Geometry: final body of the model. Coordinates: model frame, mm. Face numbers are marked on the shaded views. A direction names the side the tool comes from. Coordinates: 2 decimals unless noted, no trailing zeros. Order: outer loops, then holes, each group sorted by start corner. A loop starts at its lowest first (then second) coordinate and runs counter-clockwise, first axis right, second up. Notation, with made-up numbers: M 32,68.5 L 77,68.5 A22 cw 77,77.5 Z; hole C -25.5,62.5 d8. An arc over 180 degrees is marked long. One line per question, with ' | ' between items.
from build123d import *

# Parameters (mm, degrees)
BOSS_EXTRUDE2_DEPTH             = 2.1082
BOSS_EXTRUDE3_DEPTH             = 0.9
SKETCH13_W                      = 5.200208993
SKETCH13_H                      = 1.5
BOSS_EXTRUDE4_DEPTH             = 12.7
SKETCH16_W                      = 7.09322036
SKETCH16_H                      = 1.5
BOSS_EXTRUDE5_DEPTH             = 11.8
SKETCH17_W                      = 1.5
SKETCH17_H                      = 23.6
BOSS_EXTRUDE6_DEPTH             = 38.1
BOSS_EXTRUDE7_REACH             = 53.45
BOSS_EXTRUDE8_DEPTH             = 3.0082
CUT_EXTRUDE1_DEPTH              = 52.450131959
CUT_EXTRUDE2_REACH              = 52.338
SKETCH21_R                      = 2.794
SKETCH22_R                      = 4.572
CUT_EXTRUDE3_DEPTH              = 51.337641034
BOSS_EXTRUDE9_REACH             = 52.338
BOSS_EXTRUDE9_DIRECTION_2_DEPTH = 1.5


with BuildPart() as part:
    # Sketch6 → Boss-Extrude2 (new body)
    with BuildSketch(Plane(origin=(0, 0, 0), x_dir=(1, 0, 0), z_dir=(0, 1, 0))):
        with BuildLine():
            Line((3.1496, 3.175), (3.1496, 8.27377964))
            Line((3.1496, 8.27377964), (-5.741348421, 8.27377964))
            Line((-5.741348421, 8.27377964), (-8.59506403, 5.42006403))
            ThreePointArc((-8.59506403, 5.42006403), (-9.283317516, 4.390019898), (-9.525, 3.175))
            Line((-9.525, 3.175), (-9.525, -1.92377964))
            Line((-9.525, -1.92377964), (-6.989909723, -1.92377964))
            Line((-6.989909723, -1.92377964), (3.1496, -1.92377964))
            Line((3.1496, -1.92377964), (3.1496, 3.175))
        make_face()
    extrude(amount=BOSS_EXTRUDE2_DEPTH)

    # Sketch7 → Boss-Extrude3 (add)
    with BuildSketch(Plane.XZ):
        with BuildLine():
            Line((-2.050608993, 1.92377964), (-2.050608993, 0.42377964))
            ThreePointArc((-2.050608993, 0.42377964), (-0.881374643, -4.411978027), (-4.017957094, -8.27377964))
            Line((-4.017957094, -8.27377964), (6.35, -8.27377964))
            ThreePointArc((6.35, -8.27377964), (11.44877964, -3.175), (6.35, 1.92377964))
            Line((6.35, 1.92377964), (-2.050608993, 1.92377964))
        make_face()
    extrude(amount=BOSS_EXTRUDE3_DEPTH)

    # Sketch10 → Revolve2 (revolve)
    with BuildSketch(Plane.XY.offset(-3.175), mode=Mode.PRIVATE) as revolve2_sk:
        with BuildLine():
            Line((-6.35, 0), (-6.35, -1.065979307))
            ThreePointArc((-6.35, -1.065979307), (-5.088839039, -0.786386653), (-4.064, 0))
            Line((-4.064, 0), (-6.35, 0))
        make_face()
    revolve(revolve2_sk.sketch.rotate(Axis((-6.35, 0, -3.175), (0, -1, 0)), 180), axis=Axis((-6.35, 0, -3.175), (0, -1, 0)))

    # Sketch13 → Boss-Extrude4 (add)
    with BuildSketch(Plane.XZ):
        with Locations((0.549495504, 1.17377964)):
            Rectangle(SKETCH13_W, SKETCH13_H)
    extrude(amount=BOSS_EXTRUDE4_DEPTH)

    # Sketch16 → Boss-Extrude5 (add)
    with BuildSketch(Plane.XZ.offset(0.9)):
        with Locations((2.80338982, -7.52377964)):
            Rectangle(SKETCH16_W, SKETCH16_H)
    extrude(amount=BOSS_EXTRUDE5_DEPTH)

    # Mirror1: part across plane


with BuildPart() as part_1:
    add(part.part)
    add(part.part.mirror(Plane(origin=(3.1496, -12.7, 1.92377964), x_dir=(0, 0, 1), z_dir=(0, 1, 0))))

    # Sketch17 → Boss-Extrude6 (add)
    with BuildSketch(Plane(origin=(3.1496, 0, 0), x_dir=(0, 0, -1), z_dir=(1, 0, 0))):
        with Locations((-1.17377964, -12.7)):
            Rectangle(SKETCH17_W, SKETCH17_H)
    extrude(amount=BOSS_EXTRUDE6_DEPTH)

    # Boss-Extrude7: up to this face of the body (flat: up to its plane)
    boss_extrude7_end = Plane(part_1.part.faces().sort_by_distance((25.033512305, -24.5, 1.184664169))[0])
    # Sketch18 → Boss-Extrude7 (add, up to the picked face)
    with BuildSketch(Plane.XZ.offset(27.5082), mode=Mode.PRIVATE) as boss_extrude7_sk1:
        Polygon((3.1496, -8.27377964), (41.2496, 0.42377964), (41.2496, 1.92377964), (3.1496, 1.92377964), align=None)
    boss_extrude7_tool1 = split(extrude(boss_extrude7_sk1.sketch, amount=-BOSS_EXTRUDE7_REACH, mode=Mode.PRIVATE), bisect_by=boss_extrude7_end, keep=Keep.BOTH, mode=Mode.PRIVATE)
    add(boss_extrude7_tool1.solids().sort_by(Axis((17.478145, -27.5082, -1.539523), (0, 1, 0)))[0])

    # Sketch19 → Boss-Extrude8 (add)
    with BuildSketch(Plane(origin=(0, 2.1082, 0), x_dir=(1, 0, 0), z_dir=(0, 1, 0))):
        Polygon((3.1496, 8.27377964), (41.2496, -0.42377964), (41.2496, -1.92377964), (3.1496, -1.92377964), align=None)
    extrude(amount=-BOSS_EXTRUDE8_DEPTH)

    # Sketch20 → Cut-Extrude1 (cut, through all)
    with BuildSketch(Plane.XZ.offset(27.5082)):
        with BuildLine():
            Line((10.03132609, -6.702802721), (3.1496, -8.27377964))
            Line((3.1496, -8.27377964), (6.35, -8.27377964))
            ThreePointArc((6.35, -8.27377964), (8.351257746, -7.864618455), (10.03132609, -6.702802721))
        make_face()
    extrude(amount=-CUT_EXTRUDE1_DEPTH, mode=Mode.SUBTRACT)

    # Sketch21 → Cut-Extrude2 (cut, up to next)
    with BuildSketch(Plane(origin=(0, 0, 0.42377964), x_dir=(-1, 0, 0), z_dir=(0, 0, -1)), mode=Mode.PRIVATE) as cut_extrude2_sk1:
        with Locations((-33.6296, -2.9718)):
            Circle(SKETCH21_R)
    cut_extrude2_tool1 = extrude(cut_extrude2_sk1.sketch, amount=-CUT_EXTRUDE2_REACH, mode=Mode.PRIVATE) & part_1.part
    # Sketch21 → Cut-Extrude2 (cut, up to next)
    with BuildSketch(Plane(origin=(0, 0, 0.42377964), x_dir=(-1, 0, 0), z_dir=(0, 0, -1)), mode=Mode.PRIVATE) as cut_extrude2_sk2:
        with Locations((-13.3096, -2.9718)):
            Circle(SKETCH21_R)
    cut_extrude2_tool2 = extrude(cut_extrude2_sk2.sketch, amount=-CUT_EXTRUDE2_REACH, mode=Mode.PRIVATE) & part_1.part
    add(cut_extrude2_tool1.solids().sort_by_distance((33.6296, -2.9718, 0.42378))[0], mode=Mode.SUBTRACT)
    add(cut_extrude2_tool2.solids().sort_by_distance((13.3096, -2.9718, 0.42378))[0], mode=Mode.SUBTRACT)

    # Sketch22 → Cut-Extrude3 (cut, through all)
    with BuildSketch(Plane(origin=(0, 0, 0.42377964), x_dir=(-1, 0, 0), z_dir=(0, 0, -1))):
        with Locations((-33.6296, -2.9718)):
            Circle(SKETCH22_R)
        with Locations((-13.3096, -2.9718)):
            Circle(SKETCH22_R)
    extrude(amount=CUT_EXTRUDE3_DEPTH, mode=Mode.SUBTRACT)

    # Boss-Extrude9: up to this plane
    boss_extrude9_end = Plane(origin=(3.1496, 14.941098048, -8.27377964), z_dir=(0.2225570001625305, 0, -0.9749196796037383))
    # Sketch23 → Boss-Extrude9 (add, up to the surface)
    with BuildSketch(Plane(origin=(0, 0, 0.42377964), x_dir=(-1, 0, 0), z_dir=(0, 0, -1)), mode=Mode.PRIVATE) as boss_extrude9_sk1:
        with BuildLine():
            ThreePointArc((-29.8196, 2.1082), (-33.6296, 3.3782), (-37.4396, 2.1082))
            Line((-37.4396, 2.1082), (-29.8196, 2.1082))
        make_face()
    boss_extrude9_tool1 = split(extrude(boss_extrude9_sk1.sketch, amount=BOSS_EXTRUDE9_REACH, mode=Mode.PRIVATE), bisect_by=boss_extrude9_end, keep=Keep.BOTH, mode=Mode.PRIVATE)
    add(boss_extrude9_tool1.solids().sort_by_distance((33.6296, 2.620823, 0.42378))[0])
    # Sketch23 → Boss-Extrude9 (add, up to the surface)
    with BuildSketch(Plane(origin=(0, 0, 0.42377964), x_dir=(-1, 0, 0), z_dir=(0, 0, -1)), mode=Mode.PRIVATE) as boss_extrude9_sk2:
        with BuildLine():
            ThreePointArc((-9.4996, 2.1082), (-13.3096, 3.3782), (-17.1196, 2.1082))
            Line((-17.1196, 2.1082), (-9.4996, 2.1082))
        make_face()
    boss_extrude9_tool2 = split(extrude(boss_extrude9_sk2.sketch, amount=BOSS_EXTRUDE9_REACH, mode=Mode.PRIVATE), bisect_by=boss_extrude9_end, keep=Keep.BOTH, mode=Mode.PRIVATE)
    add(boss_extrude9_tool2.solids().sort_by_distance((13.3096, 2.620823, 0.42378))[0])

    # Sketch23 → Boss-Extrude9 direction 2 (add)
    with BuildSketch(Plane(origin=(0, 0, 0.42377964), x_dir=(-1, 0, 0), z_dir=(0, 0, -1))):
        with BuildLine():
            ThreePointArc((-29.8196, 2.1082), (-33.6296, 3.3782), (-37.4396, 2.1082))
            Line((-37.4396, 2.1082), (-29.8196, 2.1082))
        make_face()
        with BuildLine():
            ThreePointArc((-9.4996, 2.1082), (-13.3096, 3.3782), (-17.1196, 2.1082))
            Line((-17.1196, 2.1082), (-9.4996, 2.1082))
        make_face()
    extrude(amount=-BOSS_EXTRUDE9_DIRECTION_2_DEPTH)


solid = part_1.part
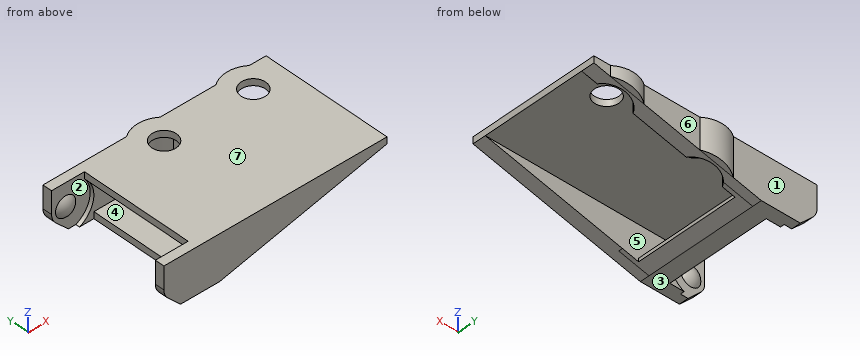
1. Section D-D, the plane y = -4.5. Output: boundary loops of the cut face in (x, z).
Response values:
outline: M -2.05,0.42 L 10.97,0.42 L 10.97,1.92 L -2.05,1.92 Z; M -0.74,-8.27 L 3.15,-8.27 L 6.35,-7.54 L 6.35,-6.77 L -0.74,-6.77 Z; M 15.65,0.42 L 31.29,0.42 L 31.29,1.92 L 15.65,1.92 Z; M 35.97,0.42 L 41.25,0.42 L 41.25,1.92 L 35.97,1.92 Z
2. Draft query along Z for the marked faces 4, 5, 6 and 7. Return one class per face: pulls with the +Z half, pulls with the -Z half, needs draft (parallel to the pull), parting line crosses it, or undercut.
Response values:
face 4: undercut | face 5: undercut | face 6: needs draft | face 7: pulls with the +Z half
3. Section A-A, the plane y = -13.5. Output: boundary loops of the cut face in (x, z).
Response values:
outline: M -2.05,0.42 L 41.25,0.42 L 41.25,1.92 L -2.05,1.92 Z; M -0.74,-8.27 L 3.15,-8.27 L 6.35,-7.54 L 6.35,-6.77 L -0.74,-6.77 Z
4. Access query for the marked faces 1, 2 and 3. Directions: +Z, -Z, +X, -X, +Y, -Y. A direction counts if a zero-diameter tool reaches every point of the face in a straight line with its end or side. Return the directions, or none.
Response values:
face 1: +Z, -Z, -X, +Y | face 2: none | face 3: -Z, +X, -X, +Y, -Y
5. Section C-C, the plane z = -6. Output: boundary loops of the cut face in (x, y).
Response values:
outline: M -8.02,-27.51 L 13.11,-27.51 L 13.11,-24.5 L -1.51,-24.5 L -1.51,-25.4 L -8.02,-25.4 Z; M -8.02,0 L -1.51,0 L -1.51,-0.9 L 9.23,-0.9 A4.57 cw 13.11,1.6 L 13.11,3.38 A6.35 ccw 9.5,2.11 L -8.02,2.11 Z
6. Section B-B, the plane x = 14.5. Output: boundary loops of the cut face in (y, z), and give its area (3 significant figures).
Response values:
outline: M -27.51,-5.68 L -24.5,-5.68 L -24.5,0.42 L -5.5,0.42 L -5.5,1.92 L -27.51,1.92 Z; M -0.44,0.42 L 1.44,0.42 L 1.44,-5.68 L 3.27,-5.68 L 3.27,1.92 L -0.44,1.92 Z | area: 68.1 mm^2
7. Material intervals for line 1 (Z direction, x = 0, y = -22.5); line 2 (Y direction, x = -3.5, z = -5.5); line 3 (Y direction, x = 25, z = -1.5), sorted ascending. Write a range as [from, to].
Response values:
line 1: z = [-8.27, -6.77], [0.42, 1.92] | line 2: y = [-27.51, -25.4], [0, 2.11] | line 3: y = [-27.51, -24.5], [-0.9, 2.11]
8. Pin query (flat end, axial travel): P1, Ø0.8, axis at y = -16, z = -7, coming from the -X side; P2, Ø4.5, axis at x = 19.5, z = -5.5, coming from the +Y side; P3, Ø5, axis at x = 20, y = -9, coming from the -Z side. Return the tip coordinate at first contact, or that it passes through.
Response values:
P1: stops at x = -0.74 | P2: stops at y = 2.11 | P3: stops at z = 0.42
